CAD build for the part. Positions are in the model's coordinates, mm. A direction names the side the tool comes from. Give positions to 0.01 mm unless a question says otherwise; leave off trailing zeros. Order: outer loops, then holes, each group sorted by start corner. A loop starts at its lowest first (then second) coordinate and runs counter-clockwise, first axis right, second up.
Item 1: Band-saw the part on A-A on y = 4. Give the cut face in (x, z).
Item 2: Band-saw the part on C-C on z = 2.75. Give the cut face in (x, y).
Item 3: Flat gauge pin, fed straight in: P1, Ø5, axis at y = -1, z = 3, coming from the -X side. Where does the tip first touch, or does it go through?
Item 4: Wall check: L1, parallel to Y at x = 2.5, z = -3.25; L2, parallel to Z at x = -2, y = 1.5; L3, parallel to Z at x = 0, y = -0.25 (3 decimals). Give the ranges that are in metal, low to high.
Item 5: Band-saw the part on B-B on x = 0.25. Give the cut face in (y, z).
Item 6: Which spindle directions (+Z, -Z, +X, -X, +Y, -Y) get a long thin tool onto all of the face, cutting with end or side? Do faces 5 (the conical face through (2.65, 5.84, 4.63)), 6 (the flat face through (-4, 0, -1)). Say none if no direction does.
Item 7: Two-plate mould, pull along X, no slides. Class faces 1 (the flat face through (-0.5, 3, 4.5)), 2 (the flat face through (0.5, 3, 4.5)), 3 (the conical face through (2.65, 0.16, 4.63)), 4 (the flat face through (0, -2.5, -2)): released by +X, released by -X, zero draft, split by the parting line, or undercut.
```python
from build123d import *

# Parameters (mm, degrees)
BOSS_EXTRUDE1_DEPTH = 6
SKETCH3_R           = 3.555
BOSS_EXTRUDE3_DEPTH = 2.5
SKETCH4_R           = 2.5
CUT_EXTRUDE1_DEPTH  = 9.5
CUT_EXTRUDE2_DEPTH  = 7


with BuildPart() as part:
    # Sketch1 → Boss-Extrude1 (new body)
    with BuildSketch(Plane(origin=(0, 0, 0), x_dir=(1, 0, 0), z_dir=(0, 1, 0))):
        Polygon((5.773502692, 0), (2.886751346, 5), (-2.886751346, 5), (-5.773502692, 0), (-2.886751346, -5), (2.886751346, -5), align=None)
    extrude(amount=BOSS_EXTRUDE1_DEPTH)

    # Sketch3 → Boss-Extrude3 (add)
    with BuildSketch(Plane.XZ):
        Circle(SKETCH3_R)
    extrude(amount=BOSS_EXTRUDE3_DEPTH)

    # Sketch4 → Cut-Extrude1 (cut, through all)
    with BuildSketch(Plane(origin=(0, 6, 0), x_dir=(1, 0, 0), z_dir=(0, 1, 0))):
        with Locations((0, -0.79)):
            Circle(SKETCH4_R)
    extrude(amount=-CUT_EXTRUDE1_DEPTH, mode=Mode.SUBTRACT)

    # Sketch5 → Cut-Extrude2 (cut, through all)
    with BuildSketch(Plane(origin=(0, 0, 0), x_dir=(-1, 0, 0), z_dir=(0, -1, 0))):
        Polygon((-1, -5), (1, -5), (0, -4), align=None)
    extrude(amount=-CUT_EXTRUDE2_DEPTH, mode=Mode.SUBTRACT)

    # Sketch6 → Cut-Revolve1 (revolve, cut)
    with BuildSketch(Plane.XY):
        Polygon((5.173502692, 6), (5.773502692, 6), (5.773502692, 5.4), align=None)
        Polygon((5.773502692, 0.6), (5.173502692, 0), (5.773502692, 0), align=None)
    revolve(axis=Axis((0, 0, 0), (0, 1, 0)), mode=Mode.SUBTRACT)


solid = part.part
```
The answers:
1. outline: (-5.77, 0) - (-2.89, -5) - (2.89, -5) - (5.77, 0) - (2.89, 5) - (1, 5) - (0, 4) - (-1, 5) - (-2.89, 5) - close; hole circle Ø5 at (0, 0.79)
2. outline: (-4.19, 0) - (-2.25, 0) - (-2.25, -2.5) - (-1.55, -2.5) - (-1.55, 6) - (-4.19, 6) - close; (1.55, -2.5) - (2.25, -2.5) - (2.25, 0) - (4.19, 0) - (4.19, 6) - (1.55, 6) - close
3. P1: stops at x = -5.31
4. L1: y = 0 to 6
4. L2: z = -5 to -0.71, 2.29 to 5
4. L3: z = -3.555 to -1.71, 3.29 to 3.555
5. outline: (-2.5, -3.55) - (0, -3.55) - (0, -5) - (6, -5) - (6, -1.7) - (-2.5, -1.7) - close; (-2.5, 3.28) - (6, 3.28) - (6, 4.25) - (0, 4.25) - (0, 3.55) - (-2.5, 3.55) - close
6. face 5: +Z, +X, +Y
6. face 6: -Y
7. face 1: undercut
7. face 2: undercut
7. face 3: released by +X
7. face 4: zero draft
